The listing builds one solid part. Answer for the finished solid, in the listing's coordinates (mm). Face numbers are marked on the shaded views. A direction names the side the tool comes from. Coordinates: 2 decimals unless noted, no trailing zeros. Order: outer loops, then holes, each group sorted by start corner. A loop starts at its lowest first (then second) coordinate and runs counter-clockwise, first axis right, second up. Notation, with made-up numbers: (48.25, 61) -> (81.25, 61) arc R12 ccw to (81.25, 72) -> close; hole circle Ø5 at (-20, 33.5). An arc over 180 degrees is marked (long way). Return JSON: item names as keys, results as strings.
Autodesk Inventor part; units mm, degrees
ref_plane "YZ Plane" through (0, 0, 0) normal (1, 0, 0) x (0, 1, 0)
ref_plane "XZ Plane" through (0, 0, 0) normal (0, 1, 0) x (-1, 0, 0)
ref_plane "XY Plane" through (0, 0, 0) normal (0, 0, 1) x (1, 0, 0)
sketch "Sketch1" plane through (0, 0, 0) normal (0, 0, 1) x (1, 0, 0)
  line L0 (0, 0) -> (150, 0)
  line L1 (150, 0) -> (150, 75)
  line L2 (150, 75) -> (0, 75)
  line L3 (0, 75) -> (0, 0)
  dimension "d0" = 150
  dimension "d1" = 75
extrude "Extrusion1" add sketch "Sketch1" along normal blind 100
chamfer "Chamfer1" distance 25 angle 45 1 edges at (150, 0, 50)
sketch "Sketch2" plane through (0, 0, 0) normal (0, -1, 0) x (1, 0, 0)
  line L0 (125, 100) -> (0, 100)
  line L1 (0, 0) -> (0, 100)
  point P0 (50, 75)
  dimension "d7" = 25
  dimension "d8" = 50
hole "Hole1" at (50, 0, 75) direction (0, 1, 0) diameter 25 end through all
sketch "Sketch3" plane through (0, 0, 0) normal (0, -1, 0) x (1, 0, 0)
  line L0 (75, 40) -> (50, 40)
  line L1 (50, 40) -> (50, 15)
  line L2 (50, 15) -> (75, 15)
  line L3 (75, 15) -> (75, 40)
  line L4 (125, 100) -> (125, 0)
  circle A0 centre (50, 75) radius 12.5
  dimension "d16" = 25
  dimension "d17" = 50
  dimension "d18" = 35
extrude "Extrusion2" cut sketch "Sketch3" against normal through all contours L3 L2 L1 L0
fillet "Fillet1" radius 3 4 edges at (50, 37.5, 15) (75, 37.5, 15) (50, 37.5, 40) (75, 37.5, 40)
chamfer "Chamfer2" distance 5 angle 45 1 edges at (50, 0, 87.5)
properties part number "pc01"
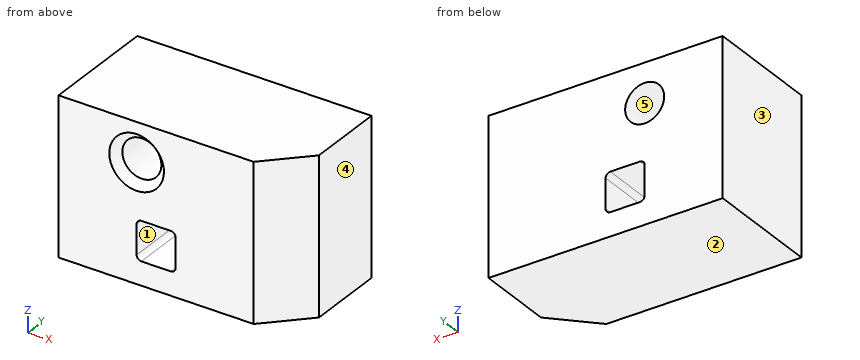
1. Each of these flat-tipped pins is pushed along its axis until it touches: pin 1 Ø1 at (x, z) = (130.5, 59.5) entering from -Y; pin 2 Ø12 at (y, z) = (9.5, 83.5) entering from +X; pin 3 Ø4 at (y, z) = (20, 58) entering from +X. Where does it stop, or does it pass through?
Answer block:
{"pin 1": "stops at y = 5", "pin 2": "stops at x = 140.5", "pin 3": "stops at x = 147"}
2. The part is cut by section C-C on z = 42. Give the vertices of the cut face in (x, y).
Answer block:
{"outline": "(0, 0) -> (125, 0) -> (150, 25) -> (150, 75) -> (0, 75) -> close"}
3. For the marked faces 1 and 2, determine the directions among +Z, -Z, +X, -X, +Y, -Y from which every point of the face is accessible in a straight line to the end or side of a thin tool.
Answer block:
{"face 1": "+Y, -Y", "face 2": "-Z, +X, -X, +Y, -Y"}
4. The part is cut by section B-B on y = 7. Give the vertices of the cut face in (x, z).
Answer block:
{"outline": "(0, 0) -> (132, 0) -> (132, 100) -> (0, 100) -> close; hole circle Ø25 at (50, 75); hole (50, 18) arc R3 ccw to (53, 15) -> (72, 15) arc R3 ccw to (75, 18) -> (75, 37) arc R3 ccw to (72, 40) -> (53, 40) arc R3 ccw to (50, 37) -> close"}
5. The part is cut by section D-D on y = 32.5. Give the vertices of the cut face in (x, z), and give its area (3 significant figures).
Answer block:
{"outline": "(0, 0) -> (150, 0) -> (150, 100) -> (0, 100) -> close; hole circle Ø25 at (50, 75); hole (50, 18) arc R3 ccw to (53, 15) -> (72, 15) arc R3 ccw to (75, 18) -> (75, 37) arc R3 ccw to (72, 40) -> (53, 40) arc R3 ccw to (50, 37) -> close", "area": "13,900 mm2"}
6. The part is cut by section A-A on z = 75. Give the vertices of the cut face in (x, y), and give its area (3 significant figures).
Answer block:
{"outline": "(0, 0) -> (32.5, 0) -> (37.5, 5) -> (37.5, 75) -> (0, 75) -> close; (62.5, 5) -> (67.5, 0) -> (125, 0) -> (150, 25) -> (150, 75) -> (62.5, 75) -> close", "area": "9,040 mm2"}
7. Consider line 1 (X direction, y = 58, z = 22); line 2 (X direction, y = 32.5, z = 75); line 3 (Z direction, x = 74.5, y = 48). Determine where each line is inside the solid, lowest interval first. Write a range as from..to.
Answer block:
{"line 1": "x = 0..50, 75..150", "line 2": "x = 0..37.5, 62.5..150", "line 3": "z = 0..16.34, 38.66..100"}
8. Determine the mould class of the marked faces 3, 4 and 5 for opening direction X: pulls with the +X half, pulls with the -X half, needs draft (parallel to the pull), parting line crosses it, or undercut.
Answer block:
{"face 3": "pulls with the -X half", "face 4": "pulls with the +X half", "face 5": "undercut"}
